Geometry check sheet. Reference: drawing and pictorial views, mm from the part's lowest x, y, z. A direction names the side the tool comes from. Round coordinates to 2 decimals unless told otherwise and drop trailing zeros. Order: outer loops, then holes, each group sorted by start corner. A loop starts at its lowest first (then second) coordinate and runs counter-clockwise, first axis right, second up.
Q1. Cross-section at A-A on z = 38. Record the cut outline in (x, y), then the cut area to 3 significant figures.
Q2. Cross-section at C-C on x = 16. Record the cut outline in (y, z).
Q3. Depth check by flat-ended pin: P1, Ø4, axis at x = 113.5, y = 88, coming from the +Z side; P2, Ø1, axis at y = 52.5, z = 38.5, coming from the +X side; P3, Ø20, axis at x = 164, z = 43, coming from the +Y side; P4, Ø8, axis at x = 100, z = 9.5, coming from the -Y side. Enter the tip coordinate at first touch or a pass-through.
Q4. Scan lines: probe 1 along Z at (x, y) = (56.5, 101.5); probe 2 along Y at (x, z) = (175, 36); probe 3 along X at (y, z) = (54, 32). Record each from-to range of solid material in increasing order.
Q5. Cross-section at B-B on y = 60. Record the cut outline in (x, z).
Q6. Set-up check for the marked faces 1, 2, 3 and 4: record each of +Z, -Z, +X, -X, +Y, -Y from which the full face is reachable in a straight line by a thin tool's end or side.
Q7. Cross-section at D-D on x = 38.5. Record the cut outline in (y, z).
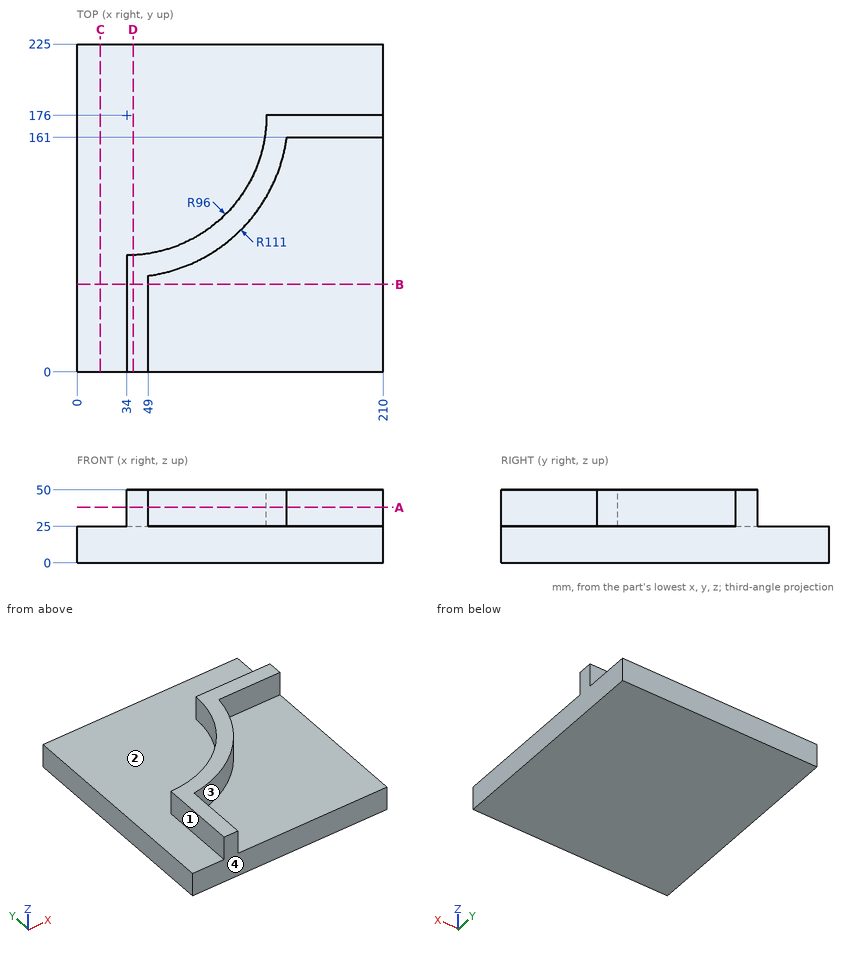
Results found:
1. outline: (34, 0) - (49, 0) - (49, 66.02) arc R111 ccw to (143.98, 161) - (210, 161) - (210, 176) - (130, 176) arc R96 cw to (34, 80) - close
1. area: 4,400 mm2
2. outline: (0, 0) - (225, 0) - (225, 25) - (0, 25) - close
3. P1: stops at z = 25
3. P2: stops at x = 49
3. P3: stops at y = 176
3. P4: stops at y = 0
4. probe 1: z = 0 to 25
4. probe 2: y = 161 to 176
4. probe 3: x = 34 to 49
5. outline: (0, 0) - (210, 0) - (210, 25) - (49, 25) - (49, 50) - (34, 50) - (34, 25) - (0, 25) - close
6. face 1: +Z, -X, +Y, -Y
6. face 2: +Z, -X, +Y
6. face 3: +Z, +X, -Y
6. face 4: +Z, -Z, +X, -X, -Y
7. outline: (0, 0) - (225, 0) - (225, 25) - (80.11, 25) - (80.11, 50) - (0, 50) - close
